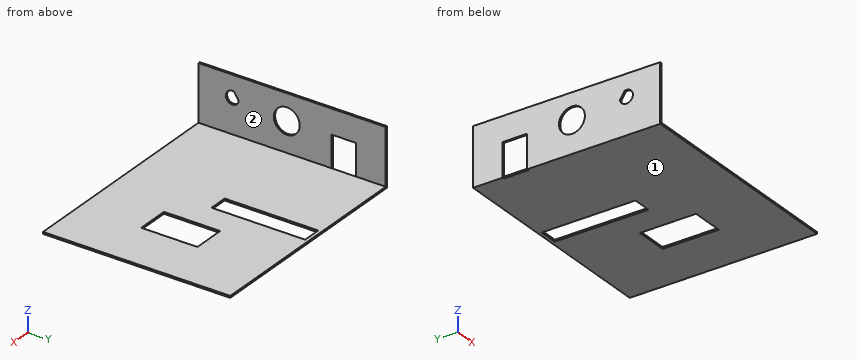
```python
from build123d import *

# Parameters (mm, degrees)
F0_W      = 304.8
F0_H      = 254
F1_DEPTH  = 2.54
F2_W      = 2.54
F2_H      = 254
F3_DEPTH  = 76.2
F4_W      = 32.960277
F4_H      = 45.472592
F5_DEPTH  = 2.54
F6_R      = 17.569994
F7_DEPTH  = 25.4
F9_DEPTH  = 25.4
F10_W     = 25.4
F10_H     = 127
F10_W_2   = 44.169486
F10_H_2   = 76.2
F11_DEPTH = 25.4


with BuildPart() as f1:
    # F0 (on Top) → F1 (new body)
    with BuildSketch(Plane.XY):
        Rectangle(F0_W, F0_H)
    extrude(amount=F1_DEPTH)

    # F2 (on face) → F3 (join)
    with BuildSketch(Plane.XY.offset(2.54)):
        with Locations((-151.13, 0)):
            Rectangle(F2_W, F2_H)
    extrude(amount=F3_DEPTH)

    # F4 (on face) → F5 (cut)
    with BuildSketch(Plane(origin=(-152.4, 0, 0), x_dir=(0, -1, 0), z_dir=(-1, 0, 0))):
        with Locations((-70.221598, 22.736296)):
            Rectangle(F4_W, F4_H)
    extrude(amount=-F5_DEPTH, mode=Mode.SUBTRACT)

    # F6 (on face) → F7 (cut)
    with BuildSketch(Plane(origin=(-152.4, 0, 0), x_dir=(0, -1, 0), z_dir=(-1, 0, 0))):
        with Locations((7.203376, 43.230873)):
            Circle(F6_R)
    extrude(amount=-F7_DEPTH, mode=Mode.SUBTRACT)

    # F8 (on face) → F9 (cut)
    with BuildSketch(Plane.YZ.offset(-149.86)):
        Polygon((-74.678751, 42.898838), (-72.551889, 46.301815), (-72.340945, 48.215244), (-78.74044, 57.646077), (-78.632851, 57.719084), (-80.081942, 58.222244), (-84.068573, 57.76337), (-87.461306, 55.620204), (-89.588167, 52.217227), (-90.027907, 48.22844), (-88.693429, 44.443871), (-85.849043, 41.613101), (-82.058114, 40.296798), (-78.071483, 40.755672), align=None)
    extrude(amount=-F9_DEPTH, mode=Mode.SUBTRACT)

    # F10 (on face) → F11 (cut)
    with BuildSketch(Plane.XY.offset(2.54)):
        with Locations((-12.7, 58.855257)):
            Rectangle(F10_W, F10_H)
        with Locations((60.076818, -4.644743)):
            Rectangle(F10_W_2, F10_H_2)
    extrude(amount=-F11_DEPTH, mode=Mode.SUBTRACT)


solid = f1.part
```
Verification items for the finished model (mm, model axes). Face numbers are marked on the shaded views. A direction names the side the tool comes from. Round coordinates to 2 decimals unless told otherwise and drop trailing zeros. Order: outer loops, then holes, each group sorted by start corner. A loop starts at its lowest first (then second) coordinate and runs counter-clockwise, first axis right, second up. Notation, with made-up numbers: (87, 70.5) -> (121, 70.5) arc R14 ccw to (121, 92.5) -> close; hole circle Ø3 at (40, 34). An arc over 180 degrees is marked (long way). Put each result on its own line as item: value. Start each with the question number.
(1) Section check B-B (y = 107.5). Enter the section's corners in (x, z).
(2) Tool access check on the marked faces 1 and 2. Record the directions out of +Z, -Z, +X, -X, +Y, -Y that give a thin tool (end or side, any length) a straight path to the whole face; none if there is none.
(3) Depth check by flat-ended pin: pin 1 Ø3 at (x, y) = (-151.5, 66) entering from -Z; pin 2 Ø5 at (x, y) = (-1.5, -72) entering from -Z; pin 3 Ø12 at (x, y) = (119.5, 88.5) entering from +Z; pin 4 Ø23 at (y, z) = (-21, 35) entering from +X. Enter the tip coordinate at first touch or a pass-through.
(4) Material ranges on line 1 along X through (y, z) = (8, 7); line 2 along Z through (x, y) = (-19, -107.5), recorded low to high.
(5) Section check A-A (z = 21). Enter the section's corners in (x, y), then the cut area to 3 significant figures.
(6) Section check D-D (y = 68). Enter the section's corners in (x, z).
(7) Section check C-C (x = 53). Enter the section's corners in (y, z), then the cut area to 3 significant figures.
Completed:
1. outline: (-152.4, 0) -> (-25.4, 0) -> (-25.4, 2.54) -> (-149.86, 2.54) -> (-149.86, 78.74) -> (-152.4, 78.74) -> close; (0, 0) -> (152.4, 0) -> (152.4, 2.54) -> (0, 2.54) -> close
2. face 1: -Z, +X, -X, +Y, -Y
2. face 2: +Z, +X, +Y, -Y
3. pin 1: stops at z = 45.47
3. pin 2: stops at z = 0
3. pin 3: stops at z = 2.54
3. pin 4: stops at x = -149.86
4. line 1: x = -152.4 to -149.86
4. line 2: z = 0 to 2.54
5. outline: (-152.4, -127) -> (-149.86, -127) -> (-149.86, 53.74) -> (-152.4, 53.74) -> close; (-152.4, 86.7) -> (-149.86, 86.7) -> (-149.86, 127) -> (-152.4, 127) -> close
5. area: 561 mm2
6. outline: (-152.4, 45.47) -> (-149.86, 45.47) -> (-149.86, 78.74) -> (-152.4, 78.74) -> close; (-149.86, 0) -> (-25.4, 0) -> (-25.4, 2.54) -> (-149.86, 2.54) -> close; (0, 0) -> (152.4, 0) -> (152.4, 2.54) -> (0, 2.54) -> close
7. outline: (-127, 0) -> (-42.74, 0) -> (-42.74, 2.54) -> (-127, 2.54) -> close; (33.46, 0) -> (127, 0) -> (127, 2.54) -> (33.46, 2.54) -> close
7. area: 452 mm2
